Input: part model. Units: mm. Frame: model coordinates. Face numbers are marked on the shaded views. A direction names the side the tool comes from. Round coordinates to 2 decimals unless told otherwise and drop trailing zeros. Loops run counter-clockwise (first coordinate to the right, second up) from the corner with the lowest first, then second, coordinate; pieces in that order, holes last.
(1) Draft query along Z for the marked faces 3, 4, 5 and 6. Return one class per face: released by +Z, released by -Z, zero draft, split by the parting line, or undercut.
(2) Line query: line 1 (Z direction, x = -35.5, y = 35.5); line 2 (X direction, y = 27, z = -41); line 3 (Z direction, x = 41, y = -49.5). Output: solid intervals per line, ascending.
(3) Access query for the marked faces 1 and 2. Directions: +Z, -Z, +X, -X, +Y, -Y. A direction counts if a zero-diameter tool reaches every point of the face in a straight line with its end or side. Return the directions, or none.
(4) First-contact query: pin 1 Ø11 at (y, z) = (128.5, -55.5) entering from +X; pin 2 Ø4 at (y, z) = (39.5, 31) entering from -X; pin 3 Ø5 at (y, z) = (107, 51) entering from -X. Flat tips, straight axial feed; report the tip coordinate or a pass-through.
(5) Cut plane D-D, the plane x = 26.5. Output: boundary loops of the cut face in (y, z), and give its area (3 significant figures).
(6) Cut plane A-A, the plane x = -29. Output: boundary loops of the cut face in (y, z), and give its area (3 significant figures).
(7) Cut plane B-B, the plane y = -16. Output: boundary loops of the cut face in (x, z).
(8) Cut plane C-C, the plane z = -32. Output: boundary loops of the cut face in (x, y).
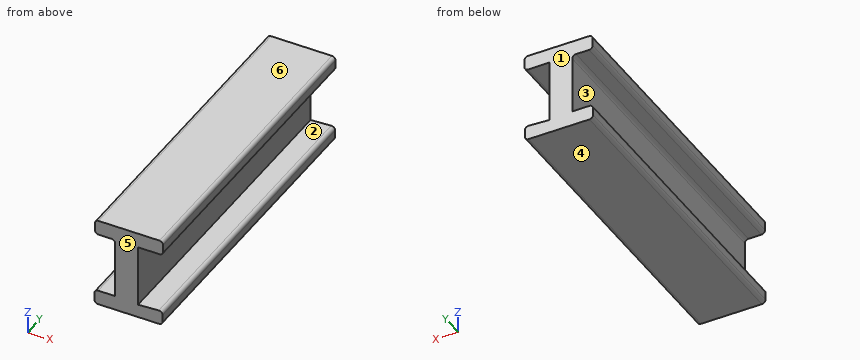
from build123d import *

# Parameters (mm, degrees)
F1_DEPTH = 76.2
F2_DEPTH = 150.114
F3_DEPTH = 209.042
F4_R     = 5.08


with BuildPart() as f1:
    # F0 (on Front) → F1 (new body)
    with BuildSketch(Plane.XZ):
        Polygon((-46.1966358125, 39.4689701498), (-18.0899463594, 39.4689701498), (-18.0899463594, -44.8510982096), (-46.7946529388, -44.8510982096), (-46.7946529388, -65.1835948229), (47.6916655898, -65.1835948229), (47.6916655898, -44.8510982096), (13.6048318818, -46.645142138), (13.6048318818, 39.7679805756), (48.2896827161, 39.4689701498), (48.2896827161, 60.1004771888), (-46.1966358125, 60.1004771888), align=None)
    extrude(amount=F1_DEPTH)

    # F2 (add): a face of the model
    f2_faces = [f1.faces().sort_by_distance(p)[0] for p in [
        (-0.6124565999, 0, -2.2518569058),
    ]]
    extrude(f2_faces, amount=F2_DEPTH)

    # F3 (add): a face of the model
    f3_faces = [f1.faces().sort_by_distance(p)[0] for p in [
        (-0.6124565999, 150.114, -2.2518569058),
    ]]
    extrude(f3_faces, amount=F3_DEPTH)

    # F4
    f4_edges = [f1.edges().sort_by_distance(p)[0] for p in [
        (-46.196636, 141.478, 39.46897),
        (-18.089946, 141.478, 39.46897),
        (-46.794653, 141.478, -44.851098),
        (-46.794653, 141.478, -65.183595),
        (47.691666, 141.478, -65.183595),
        (47.691666, 141.478, -44.851098),
        (48.289683, 141.478, 39.46897),
        (48.289683, 141.478, 60.100477),
        (-46.196636, 141.478, 60.100477),
    ]]
    fillet(f4_edges, radius=F4_R)


solid = f1.part
Reported:
1. face 3: undercut
1. face 4: released by -Z
1. face 5: zero draft
1. face 6: released by +Z
2. line 1: z = -65.18 to -44.85, 39.47 to 60.1
2. line 2: x = -18.09 to 13.6
2. line 3: z = -65.18 to -45.2, 39.53 to 60.1
3. face 1: +Z, -Z, +X, -X, +Y
3. face 2: +Y, -Y
4. pin 1: stops at x = 47.69
4. pin 2: stops at x = -18.09
4. pin 3: stops at x = -46.2
5. outline: (-76.2, -65.18) - (359.16, -65.18) - (359.16, -45.97) - (-76.2, -45.97) - close; (-76.2, 39.66) - (359.16, 39.66) - (359.16, 60.1) - (-76.2, 60.1) - close
5. area: 17,300 mm2
6. outline: (-76.2, -65.18) - (359.16, -65.18) - (359.16, -44.85) - (-76.2, -44.85) - close; (-76.2, 39.47) - (359.16, 39.47) - (359.16, 60.1) - (-76.2, 60.1) - close
6. area: 17,800 mm2
7. outline: (-46.79, -60.1) arc R5.08 ccw to (-41.71, -65.18) - (42.61, -65.18) arc R5.08 ccw to (47.69, -60.1) - (47.69, -50.21) arc R5.08 ccw to (42.34, -45.13) - (13.6, -46.65) - (13.6, 39.77) - (43.17, 39.51) arc R5.08 ccw to (48.29, 44.59) - (48.29, 55.02) arc R5.08 ccw to (43.21, 60.1) - (-41.12, 60.1) arc R5.08 ccw to (-46.2, 55.02) - (-46.2, 44.55) arc R5.08 ccw to (-41.12, 39.47) - (-23.17, 39.47) arc R5.08 cw to (-18.09, 34.39) - (-18.09, -44.85) - (-41.71, -44.85) arc R5.08 ccw to (-46.79, -49.93) - close
8. outline: (-18.09, -76.2) - (13.6, -76.2) - (13.6, 359.16) - (-18.09, 359.16) - close
